```python
from build123d import *

# Parameters (mm, degrees)
F0_R     = 48.688201
F0_R_2   = 24.133595
F1_DEPTH = 50
F2_R     = 10


with BuildPart() as f1:
    # F0 (on Front) → F1 (new body)
    with BuildSketch(Plane.XZ):
        with Locations((-10.903678, 12.357511)):
            Circle(F0_R)
        with Locations((-10.903678, 12.357511)):
            Circle(F0_R_2, mode=Mode.SUBTRACT)
    extrude(amount=F1_DEPTH)

    # F2
    f2_edges = [f1.edges().sort_by_distance(p)[0] for p in [
        (-59.591879, 0, 12.357511),
        (-35.037273, 0, 12.357511),
        (-35.037273, -50, 12.357511),
        (13.229917, -25, 12.357511),
        (-59.591879, -50, 12.357511),
    ]]
    fillet(f2_edges, radius=F2_R)


solid = f1.part
```
Part model, mm, in its own coordinate system. Coordinates: 2 decimals unless noted, no trailing zeros. Write each loop counter-clockwise with the first axis right and the second up, starting at its lowest first coordinate (ties: lowest second). Pieces come first, ordered by that corner, then holes.
Item 1: Pin check, flat tips, straight feed: pin 1 (3 mm diameter, centred on x = -14, z = -11, fed in from -Y); pin 2 (5 mm diameter, centred on x = -35.5, y = -5.5, fed in from -Z); pin 3 (6 mm diameter, centred on y = -16, z = -12, fed in from -X). Stop position of each tip, or through.
Item 2: Probe line 1 (Z direction, x = -11.5, y = -21); line 2 (Z direction, x = -27, y = -29.5); line 3 (X direction, y = -11.5, z = 26.5). List the from-to ranges inside material, lowest first.
Item 3: Slice it at B-B (y = -3.5). Write the cut outline in (x, z), and give its area (3 significant figures).
Item 4: Slice it at A-A (y = -11.5). Write the cut outline in (x, z), and give its area (3 significant figures).
Item 5: Mould opens along X. For faces 1 (the face through (11.56, -24.79, -30.84)), 2 (the face through (-16.14, -24.79, -11.2)), 3 (the face through (-11, 0, -22)) say: released by +X, released by -X, zero draft, split by the parting line, or undercut.
Results found:
1. pin 1: stops at y = -44.21
1. pin 2: stops at z = -30.25
1. pin 3: stops at x = -54.66
2. line 1: z = -36.33 to -11.77, 36.48 to 61.04
2. line 2: z = -33.59 to -5.62, 30.34 to 58.31
2. line 3: x = -57.49 to -30.46, 8.65 to 35.69
3. outline: circle Ø92.58 at (-10.9, 12.36); hole circle Ø53.07 at (-10.9, 12.36)
3. area: 4,520 mm2
4. outline: circle Ø97.38 at (-10.9, 12.36); hole circle Ø48.27 at (-10.9, 12.36)
4. area: 5,620 mm2
5. face 1: split by the parting line
5. face 2: undercut
5. face 3: zero draft
